Work out the finished part from the listing and answer in its coordinate system (mm). A direction names the side the tool comes from. Give positions to 0.01 mm unless a question says otherwise; leave off trailing zeros. Write each loop counter-clockwise with the first axis right and the second up, starting at its lowest first coordinate (ties: lowest second). Pieces come first, ordered by that corner, then holes. Notation, with made-up numbers: (4, 49.5) -> (52, 49.5) arc R22 ccw to (52, 81.5) -> close; hole circle Ø11 at (16, 37). An arc over 180 degrees is marked (long way). Use a Markdown table: item, result. Add a question column.
Q1. Consider line 1 (X direction, y = 22.5, z = 97.5); line 2 (Y direction, x = 13, z = 121); line 3 (Z direction, x = 90.5, y = 7.5). Determine where each line is inside the solid, lowest interval first.
Q2. Section D-D, the plane x = -20 is taken. Give the vertices of the cut face in (y, z).
Q3. Section A-A, the plane x = -64 is taken. Give the vertices of the cut face in (y, z), plus the area to 3 significant figures.
Q4. For a pull along Z with two mould halves and no side action, classify faces 1 (the face through (-1, 0, 0)), 2 (the face through (-93.29, 28.58, 9.87)), 3 (the face through (93.986, -29.297, 9.888)) as pulls with the +Z half, pulls with the -Z half, needs draft (parallel to the pull), parting line crosses it, or undercut.
Q5. Section C-C, the plane y = 2.5 is taken. Give the vertices of the cut face in (x, z).
Q6. For faces 4 (the face through (-1, -26.5, 120)), 5 (the face through (-1, -25.5, 118)), 6 (the face through (-93.58, -28.29, 9.87)), 7 (the face through (50, -1, 120)), 8 (the face through (-94.297, -28.986, 9.888)), determine the directions among +Z, -Z, +X, -X, +Y, -Y from which every point of the face is accessible in a straight line to the end or side of a thin tool.
Q7. Section B-B, the plane z = 167 is taken. Give the vertices of the cut face in (x, y), plus the area to 3 significant figures.
Q8. Each of these flat-tipped pins is pushed along its axis until it touches: pin 1 Ø10 at (y, z) = (8, 153) entering from +X; pin 2 Ø8 at (x, y) = (-46, 12) entering from +Z; pin 3 Ø12 at (x, y) = (-78, 15) entering from +Z. Where does it stop, or does it pass through?
from build123d import *

# Parameters (mm, degrees)
F1_DEPTH = 20
F2_W     = 101.5
F2_H     = 51.5
F3_DEPTH = 200
F4_T     = -1
F5_R     = 2
F6_R     = 0.5


with BuildPart() as f1:
    # F0 (on Top) → F1 (new body)
    with BuildSketch(Plane.XY):
        with BuildLine():
            Line((80, 35), (-80, 35))
            ThreePointArc((-80, 35), (-94.1421356237, 29.1421356237), (-100, 15))
            Line((-100, 15), (-100, -15))
            ThreePointArc((-100, -15), (-94.1421356237, -29.1421356237), (-80, -35))
            Line((-80, -35), (80, -35))
            ThreePointArc((80, -35), (94.1421356237, -29.1421356237), (100, -15))
            Line((100, -15), (100, 15))
            ThreePointArc((100, 15), (94.1421356237, 29.1421356237), (80, 35))
        make_face()
    extrude(amount=F1_DEPTH)

    # F2 (on face) → F3 (join)
    with BuildSketch(Plane.XY.offset(20)):
        with Locations((-0.75, -0.75)):
            Rectangle(F2_W, F2_H)
    extrude(amount=F3_DEPTH)

    # F4
    f4_openings = [f1.faces().sort_by_distance(p)[0] for p in [
        (-0.75, -0.75, 220),
    ]]
    offset(amount=F4_T, openings=f4_openings, kind=Kind.INTERSECTION)

    # F5
    f5_edges = [f1.edges().sort_by_distance(p)[0] for p in [
        (94.142136, -29.142136, 20),
        (100, 0, 20),
        (94.142136, 29.142136, 20),
        (0, -35, 20),
        (0, 35, 20),
        (-94.142136, -29.142136, 20),
        (-94.142136, 29.142136, 20),
        (-100, 0, 20),
        (-0.75, 25, 20),
        (-51.5, -0.75, 20),
        (-0.75, -26.5, 20),
        (50, -0.75, 20),
        (100, 15, 10),
        (80, 35, 10),
        (94.142136, 29.142136, 0),
        (-80, 35, 10),
        (0, 35, 0),
        (-100, 15, 10),
        (-94.142136, 29.142136, 0),
        (-100, -15, 10),
        (-100, 0, 0),
        (-80, -35, 10),
        (-94.142136, -29.142136, 0),
        (80, -35, 10),
        (0, -35, 0),
    ]]
    fillet(f5_edges, radius=F5_R)

    # F6
    f6_edges = [f1.edges().sort_by_distance(p)[0] for p in [
        (-51.5, -26.5, 121),
        (-51.5, 25, 121),
        (50, -26.5, 121),
        (50, 25, 121),
    ]]
    fillet(f6_edges, radius=F6_R)


solid = f1.part
Result set:
| question | item | result |
|---|---|---|
| 1 | line 1 | x = -51.5 to -50.5, 49 to 50 |
| 1 | line 2 | y = -26.5 to -25.5, 24 to 25 |
| 1 | line 3 | z = 0 to 1, 19 to 20 |
| 2 | outline | (-35, 2) arc R2 ccw to (-33, 0) -> (33, 0) arc R2 ccw to (35, 2) -> (35, 18) arc R2 ccw to (33, 20) -> (27, 20) arc R2 cw to (25, 22) -> (25, 220) -> (24, 220) -> (24, 19) -> (34, 19) -> (34, 1) -> (-34, 1) -> (-34, 19) -> (-25.5, 19) -> (-25.5, 220) -> (-26.5, 220) -> (-26.5, 22) arc R2 cw to (-28.5, 20) -> (-33, 20) arc R2 ccw to (-35, 18) -> close |
| 3 | outline | (-35, 2) arc R2 ccw to (-33, 0) -> (33, 0) arc R2 ccw to (35, 2) -> (35, 18) arc R2 ccw to (33, 20) -> (-33, 20) arc R2 ccw to (-35, 18) -> close; hole (-34, 1) -> (34, 1) -> (34, 19) -> (-34, 19) -> close |
| 3 | area | 173 mm2 |
| 4 | face 1 | pulls with the -Z half |
| 4 | face 2 | undercut |
| 4 | face 3 | needs draft |
| 5 | outline | (-100, 2) arc R2 ccw to (-98, 0) -> (98, 0) arc R2 ccw to (100, 2) -> (100, 18) arc R2 ccw to (98, 20) -> (52, 20) arc R2 cw to (50, 22) -> (50, 220) -> (49, 220) -> (49, 19) -> (99, 19) -> (99, 1) -> (-99, 1) -> (-99, 19) -> (-50.5, 19) -> (-50.5, 220) -> (-51.5, 220) -> (-51.5, 22) arc R2 cw to (-53.5, 20) -> (-98, 20) arc R2 ccw to (-100, 18) -> close |
| 6 | face 4 | +Z, +X, -X, -Y |
| 6 | face 5 | +Z |
| 6 | face 6 | none |
| 6 | face 7 | +Z, +X, +Y, -Y |
| 6 | face 8 | +Z, -Z, -X, -Y |
| 7 | outline | (-51.5, -26) arc R0.5 ccw to (-51, -26.5) -> (49.5, -26.5) arc R0.5 ccw to (50, -26) -> (50, 24.5) arc R0.5 ccw to (49.5, 25) -> (-51, 25) arc R0.5 ccw to (-51.5, 24.5) -> close; hole (-50.5, -25.5) -> (49, -25.5) -> (49, 24) -> (-50.5, 24) -> close |
| 7 | area | 302 mm2 |
| 8 | pin 1 | stops at x = 50 |
| 8 | pin 2 | stops at z = 1 |
| 8 | pin 3 | stops at z = 20 |
